from build123d import *

# Parameters (mm, degrees)
EXTRUDE_1_DEPTH     = 2
EXTRUDE_2_DEPTH     = 2
SKETCH_3_W          = 54.00760584
SKETCH_3_H          = 17.445111018
EXTRUDE_4_DEPTH     = 54
SKETCH_4_W          = 54.00760584
SKETCH_4_H          = 8.722555509
EXTRUDE_5_DEPTH     = 2
CUT_EXTRUDE_1_DEPTH = 2
SKETCH_6_R          = 1.5
CUT_EXTRUDE_2_DEPTH = 2
SKETCH_7_R          = 1.5
CUT_EXTRUDE_3_DEPTH = 2
SKETCH_8_R          = 2
CUT_EXTRUDE_4_DEPTH = 10
SKETCH_9_R          = 2
CUT_EXTRUDE_5_DEPTH = 10
CUT_EXTRUDE_6_DEPTH = 10


with BuildPart() as part:
    # 草图1 → 凸台-拉伸1 (new body)
    with BuildSketch(Plane(origin=(0, 62.5, 0), x_dir=(1, 0, 0), z_dir=(0, 1, 0))):
        Polygon((12.40278244, -4.811222629), (-45.141204286, -4.811222629), (-45.141204286, 44.365970357), (-69.141204286, 44.365970357), (-69.141204286, -4.811222629), (-69.141204286, -92.756333647), (12.40278244, -92.756333647), align=None)
    extrude(amount=EXTRUDE_1_DEPTH)

    # 草图2 → 凸台-拉伸2 (add)
    with BuildSketch(Plane(origin=(0, 64.5, 0), x_dir=(1, 0, 0), z_dir=(0, 1, 0))):
        Polygon((12.40278244, -4.811222629), (4.40278244, -4.811222629), (4.40278244, -6.811222629), (10.40278244, -6.811222629), (10.40278244, -12.811222629), (12.40278244, -12.811222629), align=None)
        Polygon((12.40278244, -66.811222629), (10.40278244, -66.811222629), (10.40278244, -72.811222629), (4.40278244, -72.811222629), (4.40278244, -74.811222629), (12.40278244, -74.811222629), align=None)
        Polygon((-69.110275928, -74.811222629), (-69.110275928, -66.811222629), (-67.110275928, -66.811222629), (-67.110275928, -72.811222629), (-61.110275928, -72.811222629), (-61.110275928, -74.811222629), align=None)
    extrude(amount=EXTRUDE_2_DEPTH)

    # 草图3 → 凸台-拉伸4 (add)
    with BuildSketch(Plane(origin=(0, 64.5, 0), x_dir=(1, 0, 0), z_dir=(0, 1, 0))):
        with Locations((-42.106473008, -84.033778138)):
            Rectangle(SKETCH_3_W, SKETCH_3_H)
    extrude(amount=EXTRUDE_4_DEPTH)

    # 草图4 → 凸台-拉伸5 (add)
    with BuildSketch(Plane(origin=(0, 118.5, 0), x_dir=(1, 0, 0), z_dir=(0, 1, 0))):
        with Locations((-42.106473008, -88.395055893)):
            Rectangle(SKETCH_4_W, SKETCH_4_H)
    extrude(amount=EXTRUDE_5_DEPTH)

    # 草图5 → 切除-拉伸1 (cut)
    with BuildSketch(Plane(origin=(0, 64.5, 0), x_dir=(1, 0, 0), z_dir=(0, 1, 0))):
        with BuildLine():
            Line((-69.141204286, 44.365970357), (-45.141204286, 44.365970357))
            Line((-45.141204286, 44.365970357), (-45.141204286, 12.939643007))
            Line((-45.141204286, 12.939643007), (-45.141204286, -3.210429493))
            Line((-45.141204286, -3.210429493), (-52.09989667, -3.210429493))
            Line((-52.09989667, -3.210429493), (-52.09989667, 2.442121652))
            ThreePointArc((-52.09989667, 2.442121652), (-57.960262195, 8.302487177), (-63.820627721, 2.442121652))
            Line((-63.820627721, 2.442121652), (-63.820627721, -3.210429493))
            Line((-63.820627721, -3.210429493), (-69.141204286, -3.210429493))
            Line((-69.141204286, -3.210429493), (-69.141204286, 12.939643007))
            Line((-69.141204286, 12.939643007), (-69.141204286, 44.365970357))
        make_face()
    extrude(amount=-CUT_EXTRUDE_1_DEPTH, mode=Mode.SUBTRACT)

    # 草图6 → 切除-拉伸2 (cut)
    with BuildSketch(Plane(origin=(0, 64.5, 0), x_dir=(1, 0, 0), z_dir=(0, 1, 0))):
        with Locations(Location((-57.960262195, 2.065309301, 0), (0, 0, 270))):
            Circle(SKETCH_6_R)
    extrude(amount=-CUT_EXTRUDE_2_DEPTH, mode=Mode.SUBTRACT)

    # 草图7 → 切除-拉伸3 (cut)
    with BuildSketch(Plane(origin=(0, 64.5, 0), x_dir=(1, 0, 0), z_dir=(0, 1, 0))):
        with Locations(Location((2.40278244, -84.756333647, 0), (0, 0, 270))):
            Circle(SKETCH_7_R)
    extrude(amount=-CUT_EXTRUDE_3_DEPTH, mode=Mode.SUBTRACT)

    # 草图8 → 切除-拉伸4 (cut)
    with BuildSketch(Plane.XY.offset(92.756333647)):
        with Locations((-62.862887917, 103.952611989)):
            Circle(SKETCH_8_R)
        with Locations((-25.762887917, 103.952611989)):
            Circle(SKETCH_8_R)
    extrude(amount=-CUT_EXTRUDE_4_DEPTH, mode=Mode.SUBTRACT)

    # 草图9 → 切除-拉伸5 (cut)
    with BuildSketch(Plane.XY.offset(92.756333647)):
        with Locations((-25.762887917, 78.952611989)):
            Circle(SKETCH_9_R)
        with Locations((-25.762887917, 88.952611989)):
            Circle(SKETCH_9_R)
    extrude(amount=-CUT_EXTRUDE_5_DEPTH, mode=Mode.SUBTRACT)

    # 草图10 → 切除-拉伸6 (cut)
    with BuildSketch(Plane(origin=(0, 64.5, 0), x_dir=(1, 0, 0), z_dir=(0, 1, 0))):
        with BuildLine():
            Line((-49.641043763, -12.895188862), (0.358956237, -12.895188862))
            ThreePointArc((0.358956237, -12.895188862), (3.894490143, -14.359654957), (5.358956237, -17.895188862))
            Line((5.358956237, -17.895188862), (5.358956237, -37.683198524))
            ThreePointArc((5.358956237, -37.683198524), (-3.623853253, -40.587654582), (-11.606455481, -45.627971337))
            Line((-11.606455481, -45.627971337), (-52.141043763, -22.225315881))
            ThreePointArc((-52.141043763, -22.225315881), (-54.470672894, -16.601093637), (-49.641043763, -12.895188862))
        make_face()
        with BuildLine():
            Line((-20.324564628, -55.916079989), (-56.450495194, -35.058764253))
            ThreePointArc((-56.450495194, -35.058764253), (-59.11319003, -35.058764253), (-60.444537448, -37.364725623))
            Line((-60.444537448, -37.364725623), (-60.444537448, -67.07683336))
            ThreePointArc((-60.444537448, -67.07683336), (-60.004346188, -68.139549071), (-58.941630477, -68.579740332))
            Line((-58.941630477, -68.579740332), (-24.870187523, -68.579740332))
            ThreePointArc((-24.870187523, -68.579740332), (-23.165506378, -62.043979698), (-20.324564628, -55.916079989))
        make_face()
    extrude(amount=-CUT_EXTRUDE_6_DEPTH, mode=Mode.SUBTRACT)


solid = part.part
For this review, take the finished solid that the model builds, in its own axes (mm). A direction names the side the tool comes from. Round coordinates to 2 decimals unless told otherwise and drop trailing zeros. Write each loop counter-clockwise with the first axis right and the second up, starting at its lowest first coordinate (ties: lowest second). Pieces come first, ordered by that corner, then holes. Notation, with made-up numbers: (-5.5, 85) - (26.5, 85) arc R25 cw to (26.5, 99) - close; hole circle Ø6 at (-37, 76.25). An arc over 180 degrees is marked (long way). Write item = value, one per line. Start each with the question number.
1. Draft analysis for pull direction X (two halves, no side actions). For faces 1 (the face through (-59.425, 63.514, -2.39)), 2 (the face through (-15.103, 92, 84)), 3 (the face through (-29, 62.5, 42)), state which applies: released by +X, released by -X, zero draft, split by the parting line, or undercut.
2. Consider section A-A on x = -13.5. State the section outline as (y, z) points, plus the area to 3 significant figures.
3. Consider section C-C on x = -31.5. State the section outline as (y, z) points.
4. Consider section D-D on y = 73.5. State the section outline as (x, z) points, plus the area to 3 significant figures.
5. For faces 4 (the face through (-26, 79, 82.756)), 5 (the face through (-67, 66.5, 73)), 6 (the face through (3.855, 63.514, 14.321)), 7 (the face through (-16, 64, 4.811)), list the 3-axis set-ups (+Z, -Z, +X, -X, +Y, -Y) from which the entire face can be reached by the end or side of a thin tool; tool diameter is ignored.
6. Wall thickness on L1, parallel to Z at x = -42.5, y = 86; L2, parallel to X at y = 117.5, z = 77; L3, parallel to Z at x = -24, y = 104: over which ranges is each line inside the solid? List them lowest first.
7. For pin 1 Ø0.6 at (y, z) = (65, 69.5) entering from -X; pin 2 Ø0.8 at (y, z) = (63, 3.5) entering from +X; pin 3 Ø1.2 at (x, y) = (-26.5, 88.5) entering from +Z, all flat-tipped, find the tip position at first contact; note any pin that passes through.
Evaluation:
q1.face_1 = undercut
q1.face_2 = released by +X
q1.face_3 = zero draft
q2.outline = (62.5, 4.81) - (64.5, 4.81) - (64.5, 12.9) - (62.5, 12.9) - close; (62.5, 44.53) - (64.5, 44.53) - (64.5, 92.76) - (62.5, 92.76) - close
q2.area = 113 mm2
q3.outline = (62.5, 4.81) - (64.5, 4.81) - (64.5, 12.9) - (62.5, 12.9) - close; (62.5, 34.14) - (64.5, 34.14) - (64.5, 49.46) - (62.5, 49.46) - close; (62.5, 68.58) - (64.5, 68.58) - (64.5, 75.31) - (118.5, 75.31) - (118.5, 84.03) - (120.5, 84.03) - (120.5, 92.76) - (62.5, 92.76) - close
q4.outline = (-69.11, 75.31) - (-15.1, 75.31) - (-15.1, 92.76) - (-69.11, 92.76) - close
q4.area = 942 mm2
q5.face_4 = +Z
q5.face_5 = -Z, +X, -X, +Y
q5.face_6 = +Y, -Y
q5.face_7 = -Z, +X, +Y, -Y
q6.L1 = 75.31 to 92.76
q6.L2 = -69.11 to -15.1
q6.L3 = 75.31 to 82.76
q7.pin_1 = -69.11
q7.pin_2 = -45.14
q7.pin_3 = 82.76
